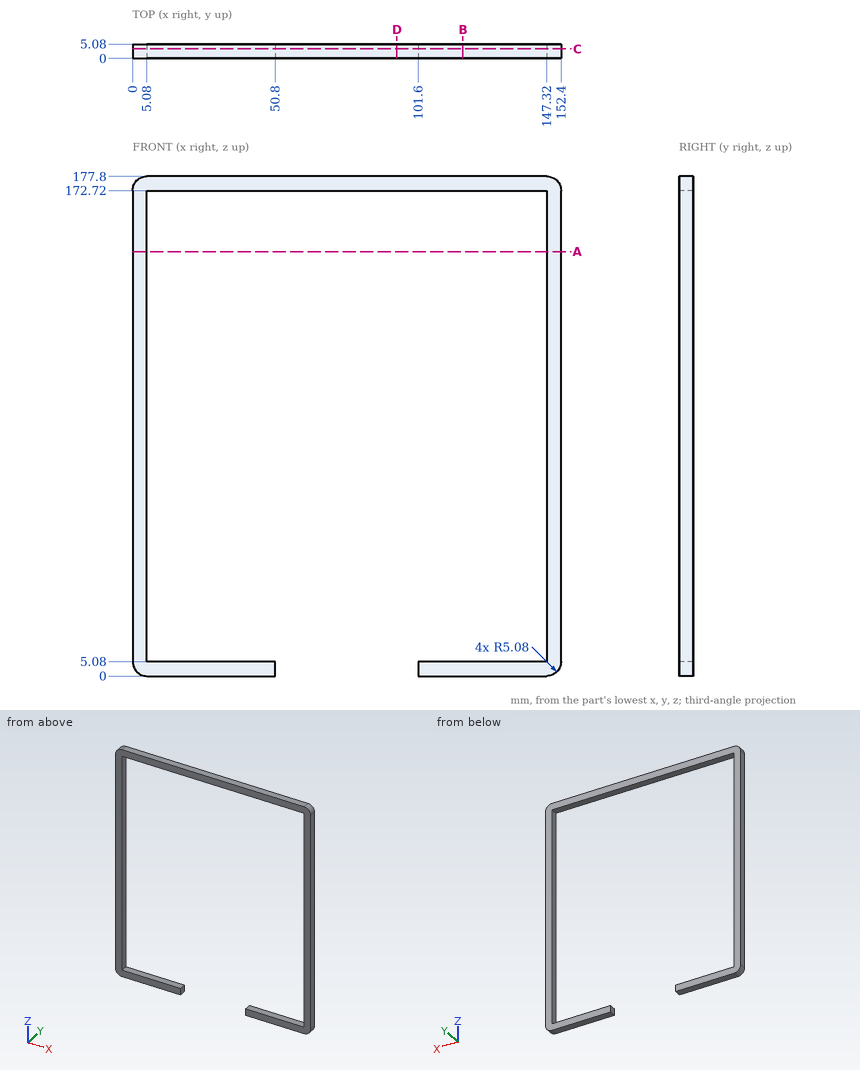
The figure shows three views and two pictorial views of one solid part (mm, origin at its lowest corner). Answer the questions. Coordinates: 2 decimals unless noted, no trailing zeros. Write each loop counter-clockwise with the first axis right and the second up, starting at its lowest first coordinate (ties: lowest second). Pieces come first, ordered by that corner, then holes. Notation, with made-up numbers: (44, -14) -> (57, -14) arc R26 ccw to (57, 9) -> close; hole circle Ø7 at (35, -32.75). An arc over 180 degrees is marked (long way). Return JSON: item names as keys, results as strings.
(1) Consider line 1 along X through (y, z) = (1.65, 162.5); line 2 along Z through (x, y) = (107, 3.65); line 3 along Z through (x, y) = (80, 2.9). Determine where each line is inside the solid, lowest interval first. Write a range as from..to.
Answers below:
{"line 1": "0..5.08, 147.32..152.4", "line 2": "0..5.08, 172.72..177.8", "line 3": "172.72..177.8"}
(2) Each of these flat-tipped pins is pushed along its axis until it touches: P1, Ø2, axis at x = 59, y = 2.5, coming from the -Z side; P2, Ø2.5, axis at y = 4, z = 2, coming from the +X side. Where does it stop, or does it pass through?
Answers below:
{"P1": "z = 172.72", "P2": "x = 152.06"}
(3) The part is cut by section C-C on y = 3.35. Give the vertices of the cut face in (x, z), then the cut area to 3 significant figures.
Answers below:
{"outline": "(0, 5.08) arc R5.08 ccw to (5.08, 0) -> (50.8, 0) -> (50.8, 5.08) -> (5.08, 5.08) -> (5.08, 172.72) -> (147.32, 172.72) -> (147.32, 5.08) -> (101.6, 5.08) -> (101.6, 0) -> (147.32, 0) arc R5.08 ccw to (152.4, 5.08) -> (152.4, 172.72) arc R5.08 ccw to (147.32, 177.8) -> (5.08, 177.8) arc R5.08 ccw to (0, 172.72) -> close", "area": "2,970 mm^2"}
(4) The part is cut by section B-B on x = 117.5. Give the vertices of the cut face in (y, z), then the cut area to 3 significant figures.
Answers below:
{"outline": "(0, 0) -> (5.08, 0) -> (5.08, 5.08) -> (0, 5.08) -> close; (0, 172.72) -> (5.08, 172.72) -> (5.08, 177.8) -> (0, 177.8) -> close", "area": "51.6 mm^2"}
(5) The part is cut by section A-A on z = 151. Give the vertices of the cut face in (x, y), then the cut area to 3 significant figures.
Answers below:
{"outline": "(0, 0) -> (5.08, 0) -> (5.08, 5.08) -> (0, 5.08) -> close; (147.32, 0) -> (152.4, 0) -> (152.4, 5.08) -> (147.32, 5.08) -> close", "area": "51.6 mm^2"}
(6) The part is cut by section D-D on x = 94. Give the vertices of the cut face in (y, z).
Answers below:
{"outline": "(0, 172.72) -> (5.08, 172.72) -> (5.08, 177.8) -> (0, 177.8) -> close"}
